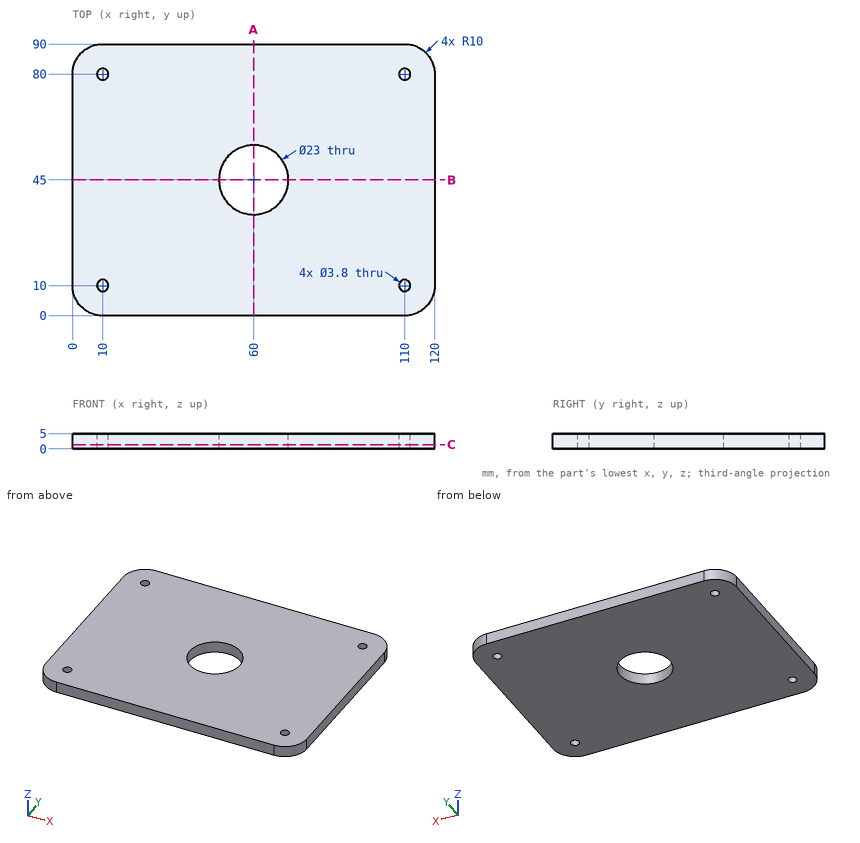
Study the drawing (mm; zero at the part's minimum x, y, z) and answer. Give positions to 0.01 mm unless a question says otherwise; leave off trailing zeros. Order: outer loops, then holes, each group sorted by start corner. A loop starts at its lowest first (then second) coordinate and runs counter-clockwise, first axis right, second up.
1. Section B-B, the plane y = 45 is taken. Determine the outline of the cut face in (x, z).
Result sheet:
outline: (0, 0) - (48.5, 0) - (48.5, 5) - (0, 5) - close; (71.5, 0) - (120, 0) - (120, 5) - (71.5, 5) - close
2. Section C-C, the plane z = 1.4 is taken. Determine the outline of the cut face in (x, y).
Result sheet:
outline: (0, 10) arc R10 ccw to (10, 0) - (110, 0) arc R10 ccw to (120, 10) - (120, 80) arc R10 ccw to (110, 90) - (10, 90) arc R10 ccw to (0, 80) - close; hole circle Ø3.8 at (10, 10); hole circle Ø3.8 at (10, 80); hole circle Ø23 at (60, 45); hole circle Ø3.8 at (110, 10); hole circle Ø3.8 at (110, 80)
3. Straight lines are drawn through the part: L1, parallel to Y at x = 10, z = 3.1; L2, parallel to Y at x = 68, z = 2.75; L3, parallel to X at y = 38, z = 2. For each, find the intervals that lie inside material, in ascending order.
Result sheet:
L1: y = 0 to 8.1, 11.9 to 78.1, 81.9 to 90
L2: y = 0 to 36.74, 53.26 to 90
L3: x = 0 to 50.88, 69.12 to 120
4. Section A-A, the plane x = 60 is taken. Determine the outline of the cut face in (y, z).
Result sheet:
outline: (0, 0) - (33.5, 0) - (33.5, 5) - (0, 5) - close; (56.5, 0) - (90, 0) - (90, 5) - (56.5, 5) - close
